Could you check a few things on this model? Use its own coordinates, in mm. Coordinates: 2 decimals unless noted, no trailing zeros. Loops run counter-clockwise (first coordinate to the right, second up) from the corner with the lowest first, then second, coordinate; pieces in that order, holes last.
1) Will these pins go through, and if not, where does the flat tip stop? P1, Ø6.5, axis at x = 7.5, z = 12.5, coming from the -Y side; P2, Ø1.8, axis at x = 6.5, y = -9, coming from the -Z side.
2) Imagine slicing it at C-C on y = 10. Please give me the cut outline in (x, z).
3) Imagine slicing it at A-A on z = 13. Please give me the cut outline in (x, y), plus the area to 3 significant figures.
4) Imagine slicing it at D-D on z = -34.5. Please give me the cut outline in (x, y), plus the area to 3 significant figures.
5) If I drill on line 1 along Z through (x, y) = (6, -12.5); line 2 along Z through (x, y) = (5.75, -13.5); line 3 along Y through (x, z) = (6, -35.25), over which ranges is the centre line in solid material (lowest first)?
6) Imagine slicing it at B-B on y = -10. Please give me the cut outline in (x, z), plus the area to 3 significant figures.
Autodesk Inventor part; units mm, degrees
ref_plane "YZ Plane" through (0, 0, 0) normal (1, 0, 0) x (0, 1, 0)
ref_plane "XZ Plane" through (0, 0, 0) normal (0, 1, 0) x (-1, 0, 0)
ref_plane "XY Plane" through (0, 0, 0) normal (0, 0, 1) x (1, 0, 0)
sketch "Sketch1" plane through (0, 0, 0) normal (1, 0, 0) x (0, 1, 0)
  line L0 (20, 43) -> (-20, 43)
  line L1 (-20, 43) -> (-20, -43)
  line L2 (-20, -43) -> (20, -43)
  line L3 (20, -43) -> (20, 43)
  line L4 (20, 43) -> (-20, -43) construction
  line L5 (-20, 43) -> (20, -43) construction
  point P0 (0, 0)
  dimension "d0" = 40
  dimension "d1" = 86
extrude "Extrusion1" add sketch "Sketch1" along normal blind 12
sketch "Sketch2" plane through (0, -20, -43) normal (0, -1, 0) x (1, 0, 0)
  circle A0 centre (6, 56) radius 3
  circle A1 centre (6, 76) radius 3
  line L0 (0, 86) -> (12, 86)
  line L1 (6, 86) -> (6, 56) construction
  point P0 (0, 43)
  dimension "d4" = 6
  dimension "d6" = 10
  dimension "d7" = 20
extrude "Extrusion2" cut sketch "Sketch2" against normal blind 15
sketch "Sketch3" plane through (0, -20, -43) normal (0, 0, -1) x (-1, 0, 0)
  line L0 (0, 40) -> (-12, 40)
  line L1 (-6, 40) -> (-6, 0) construction
  line L2 (0, 0) -> (-12, 0)
  circle A0 centre (-6, 30) radius 3
  circle A1 centre (-6, 10) radius 3
  point P0 (0, 20)
  dimension "d10" = 6
  dimension "d11" = 10
  dimension "d12" = 20
extrude "Extrusion3" cut sketch "Sketch3" against normal blind 15
thread "Thread1"
thread "Thread2"
thread "Thread3"
thread "Thread4"
properties part number "MotorHolderLongAxisTop"
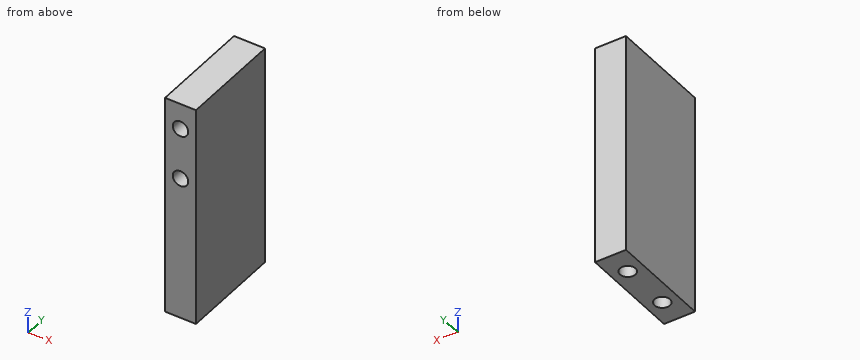
Filled in:
1. P1: stops at y = -20
1. P2: stops at z = -28
2. outline: (0, -43) - (3, -43) - (3, -28) - (9, -28) - (9, -43) - (12, -43) - (12, 43) - (0, 43) - close
3. outline: (0, -20) - (3, -20) - (3, -5) - (9, -5) - (9, -20) - (12, -20) - (12, 20) - (0, 20) - close
3. area: 390 mm2
4. outline: (0, -20) - (12, -20) - (12, 20) - (0, 20) - close; hole circle Ø6 at (6, -10); hole circle Ø6 at (6, 10)
4. area: 423 mm2
5. line 1: z = -28 to 10, 16 to 30, 36 to 43
5. line 2: z = -43 to 10.01, 15.99 to 30.01, 35.99 to 43
5. line 3: y = -20 to -13, -7 to 7, 13 to 20
6. outline: (0, -43) - (3, -43) - (3, -28) - (9, -28) - (9, -43) - (12, -43) - (12, 43) - (0, 43) - close; hole circle Ø6 at (6, 13); hole circle Ø6 at (6, 33)
6. area: 885 mm2
